Check sheet for the drawn part. Datum: minimum x, y, z corner. Units: mm. A direction names the side the tool comes from. Give positions to 0.01 mm unless a question says otherwise; leave off trailing zeros. Loops run counter-clockwise (first coordinate to the right, second up) from the corner with the lowest first, then second, coordinate; pieces in that order, holes last.
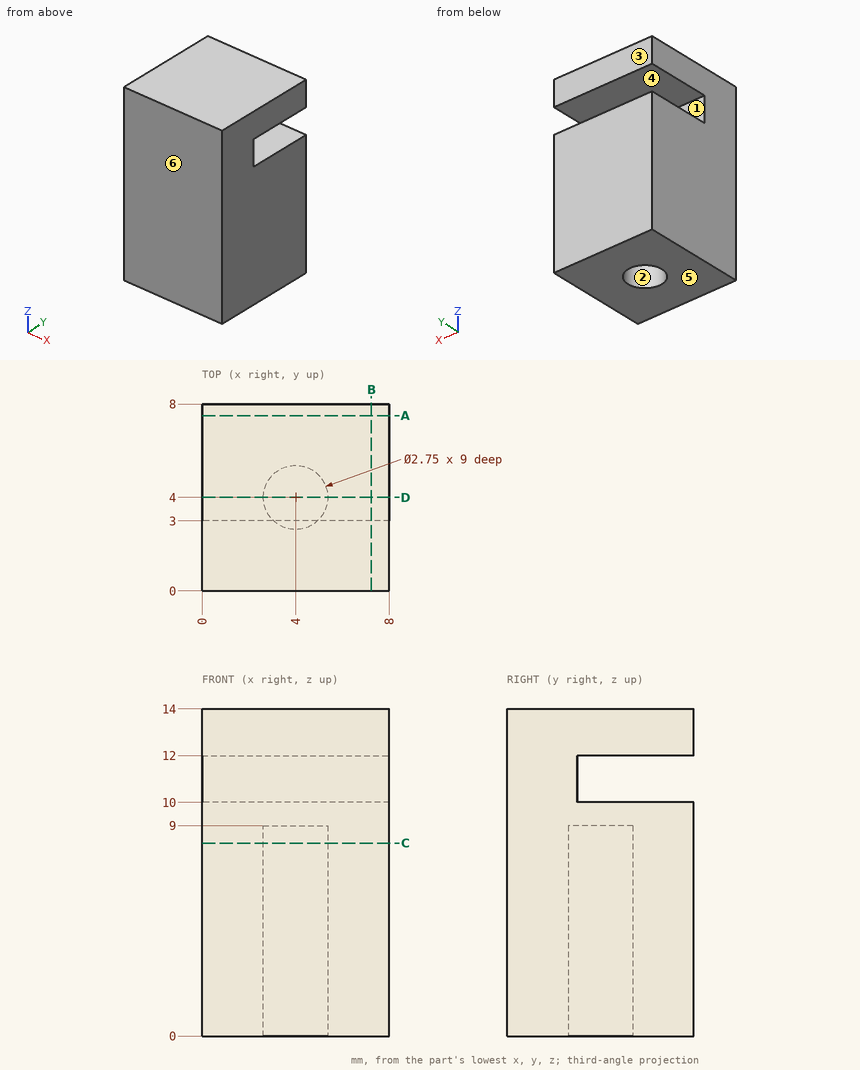
(1) Section check D-D on y = 4. Record the boundary of the cut face in (x, z) (3 decimals), plus the area to 4 significant figures.
(2) Material ranges on line 1 (Z direction, x = 3.75, y = 7.25); line 2 (Z direction, x = 3.5, y = 5); line 3 (Y direction, x = 4, z = 5.5) (3 decimals), recorded low to high.
(3) Release check for a two-part mould opening along Z. For the marked faces 4, 5 and 6 record: pulls with the +Z half, pulls with the -Z half, needs draft (parallel to the pull), parting line crosses it, or undercut.
(4) Section check C-C on z = 8.25. Record the boundary of the cut face in (x, y) (3 decimals).
(5) Section check A-A on y = 7.5. Record the boundary of the cut face in (x, z).
(6) Access from +Z, -Z, +X, -X, +Y, -Y to the whole of each face (thin tool, end or side, straight path). Record for the marked faces 1, 2 and 3.
(7) Gauge pin test, flat end, axial feed: pin 1 Ø1.6 at (x, z) = (5.5, 11) entering from +Y. Record the tip position at first contact, or that the pin passes through.
(8) Section check B-B on x = 7.25. Record the boundary of the cut face in (y, z).
Computed values:
1. outline: (0, 0) - (2.625, 0) - (2.625, 9) - (5.375, 9) - (5.375, 0) - (8, 0) - (8, 10) - (0, 10) - close; (0, 12) - (8, 12) - (8, 14) - (0, 14) - close
1. area: 71.25 mm2
2. line 1: z = 0 to 10, 12 to 14
2. line 2: z = 9 to 10, 12 to 14
2. line 3: y = 0 to 2.625, 5.375 to 8
3. face 4: undercut
3. face 5: pulls with the -Z half
3. face 6: needs draft
4. outline: (0, 0) - (8, 0) - (8, 8) - (0, 8) - close; hole circle Ø2.75 at (4, 4)
5. outline: (0, 0) - (8, 0) - (8, 10) - (0, 10) - close; (0, 12) - (8, 12) - (8, 14) - (0, 14) - close
6. face 1: +X, -X, +Y
6. face 2: -Z
6. face 3: +Z, -Z, +X, -X, +Y
7. pin 1: stops at y = 3
8. outline: (0, 0) - (8, 0) - (8, 10) - (3, 10) - (3, 12) - (8, 12) - (8, 14) - (0, 14) - close
